Can you work these out from the model? Positions are in its coordinate system, mm. Face numbers are marked on the shaded views. A direction names the side the tool comes from. Give positions to 0.01 mm unless a question says otherwise; leave off trailing zeros. Order: outer loops, then holes, each group sorted by start corner. A loop starts at its lowest first (then second) coordinate and runs counter-clockwise, first axis right, second up. Notation, with made-up numbers: M 82,26.5 L 125,26.5 A22 cw 125,34.5 Z; hole C 24,-11.75 d2. An arc over 180 degrees is marked long. One line per question, with ' | ' between items. Start each with the question number.
1) If we section it at C-C, the plane y = 24: Please give me the cut outline in (x, z).
2) Please list where these lines run through material, in increasing order: line 1 along Z through (x, y) = (147, 0.75); line 2 along X through (y, z) = (1.15, -40.5); line 3 along Z through (x, y) = (34, 52). Write a range as [from, to].
3) If we section it at A-A, the plane z = -22: Please give me the cut outline in (x, y), plus the area to 3 significant figures.
4) I'm going to push flat-ended pins straight in: pin 1 Ø10 at (x, y) = (66.5, 10) entering from +Z; pin 2 Ø4 at (y, z) = (34.5, -45) entering from -X; pin 3 Ø3.5 at (x, z) = (107.5, -44.5) entering from -Y. Where does each tip first touch, or does it pass through?
5) Thinking about a two-plate mould opening in Z: for the marked faces 1, 2 and 3, which applies, +Z half, -Z half, draft (parallel to the pull), parting line (faces both ways), or undercut?
6) If we section it at D-D, the plane x = 107.5: Please give me the cut outline in (y, z), plus the area to 3 significant figures.
7) For the marked faces 4, 5 and 6, which set-ups out of +Z, -Z, +X, -X, +Y, -Y let a thin tool reach every point of the face, with its end or its side?
8) If we section it at B-B, the plane x = 87: Please give me the cut outline in (y, z).
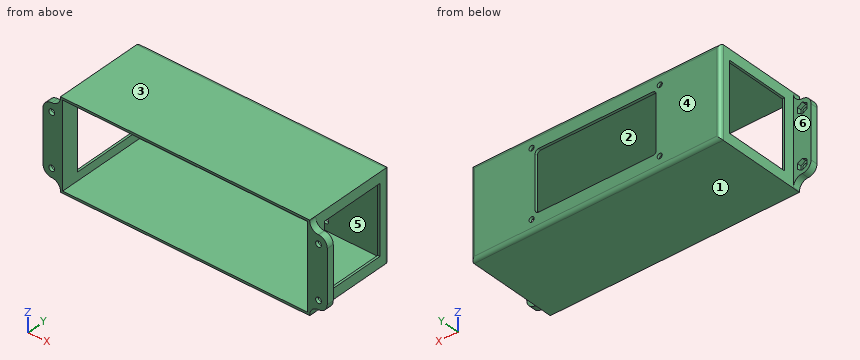
```python
from build123d import *

# Parameters (mm, degrees)
SKETCH1_W                 = 142
SKETCH1_H                 = 51
BOSS_EXTRUDE1_DEPTH       = 53
SHELL1_T                  = -1.25
SHELL1_THICKNESS_2_FACE_W = 48.5
SHELL1_THICKNESS_2_FACE_H = 139.5
SHELL1_THICKNESS_2_DEPTH  = 0.25
SKETCH2_W                 = 10
SKETCH2_H                 = 40
SKETCH2_R                 = 1.65
BOSS_EXTRUDE2_DEPTH       = 4
SKETCH3_W                 = 39
SKETCH3_H                 = 37
CUT_EXTRUDE1_DEPTH        = 169.860889492
CUT_EXTRUDE2_DEPTH        = 2.3
FILLET2_START             = -1
FILLET2_DEPTH             = 5
FILLET2_2_DEPTH           = 4
SKETCH5_R                 = 1.45
CUT_EXTRUDE3_DEPTH        = 169.860889492
SKETCH7_W                 = 69
SKETCH7_H                 = 34
CUT_EXTRUDE4_DEPTH        = 169.860889492
FILLET6_R                 = 2
FILLET7_R                 = 2


with BuildPart() as part:
    # Sketch1 → Boss-Extrude1 (new body)
    with BuildSketch(Plane(origin=(0, 0, 0), x_dir=(1, 0, 0), z_dir=(0, 1, 0))):
        with Locations((71, 25.5)):
            Rectangle(SKETCH1_W, SKETCH1_H)
    extrude(amount=BOSS_EXTRUDE1_DEPTH)

    # Shell1
    shell1_openings = [part.faces().sort_by_distance(p)[0] for p in [
        (71, 0, -25.5),
    ]]
    offset(amount=SHELL1_T, openings=shell1_openings, kind=Kind.INTERSECTION)

    # Shell1 thickness 2 face (on inner face of the shell) → Shell1 thickness 2 (add)
    with BuildSketch(Plane(origin=(71, 51.75, -25.5), x_dir=(0, 0, 1), z_dir=(0, 1, 0))):
        Rectangle(SHELL1_THICKNESS_2_FACE_W, SHELL1_THICKNESS_2_FACE_H)
    extrude(amount=-SHELL1_THICKNESS_2_DEPTH)

    # Sketch2 → Boss-Extrude2 (add)
    # profile 1 of 2: a face of its own
    with BuildSketch(Plane.XZ):
        with Locations((147, -25.5)):
            Rectangle(SKETCH2_W, SKETCH2_H)
        with Locations(Location((147, -40.5, 0), (0, 0, 270))):
            Circle(SKETCH2_R, mode=Mode.SUBTRACT)
        with Locations(Location((147, -10.5, 0), (0, 0, 270))):
            Circle(SKETCH2_R, mode=Mode.SUBTRACT)
    # profile 2 of 2: a face of its own
    with BuildSketch(Plane.XZ):
        with Locations((-5, -25.5)):
            Rectangle(SKETCH2_W, SKETCH2_H)
        with Locations(Location((-5, -40.5, 0), (0, 0, 270))):
            Circle(SKETCH2_R, mode=Mode.SUBTRACT)
        with Locations(Location((-5, -10.5, 0), (0, 0, 270))):
            Circle(SKETCH2_R, mode=Mode.SUBTRACT)
    extrude(amount=-BOSS_EXTRUDE2_DEPTH)

    # Sketch3 → Cut-Extrude1 (cut, through all)
    with BuildSketch(Plane(origin=(142, 0, 0), x_dir=(0, 0, -1), z_dir=(1, 0, 0))):
        with Locations((25.5, 28.5)):
            Rectangle(SKETCH3_W, SKETCH3_H)
    extrude(amount=-CUT_EXTRUDE1_DEPTH, mode=Mode.SUBTRACT)

    # Sketch4 → Cut-Extrude2 (cut)
    with BuildSketch(Plane(origin=(0, 4, 0), x_dir=(1, 0, 0), z_dir=(0, 1, 0))):
        Polygon((-5, 43.675426481), (-7.75, 42.08771324), (-7.75, 38.91228676), (-5, 37.324573519), (-2.25, 38.91228676), (-2.25, 42.08771324), align=None)
        Polygon((-5, 13.675426481), (-7.75, 12.08771324), (-7.75, 8.91228676), (-5, 7.324573519), (-2.25, 8.91228676), (-2.25, 12.08771324), align=None)
        Polygon((147, 43.675426481), (144.25, 42.08771324), (144.25, 38.91228676), (147, 37.324573519), (149.75, 38.91228676), (149.75, 42.08771324), align=None)
        Polygon((147, 13.675426481), (144.25, 12.08771324), (144.25, 8.91228676), (147, 7.324573519), (149.75, 8.91228676), (149.75, 12.08771324), align=None)
    extrude(amount=-CUT_EXTRUDE2_DEPTH, mode=Mode.SUBTRACT)

    # Fillet2: read off the stored shape, not the designer's step
    # Fillet2 outline → Fillet2 (cut)
    with BuildSketch(Plane(origin=(0, 0, 0), x_dir=(1, 0, 0), z_dir=(0, 1, 0)).offset(FILLET2_START)):
        with BuildLine():
            Line((-10, 5.5), (-5, 5.5))
            ThreePointArc((-5, 5.5), (-8.535533906, 6.964466094), (-10, 10.5))
            Line((-10, 10.5), (-10, 5.5))
        make_face()
        with BuildLine():
            Line((-10, 45.5), (-10, 40.5))
            ThreePointArc((-10, 40.5), (-8.535533906, 44.035533906), (-5, 45.5))
            Line((-5, 45.5), (-10, 45.5))
        make_face()
        with BuildLine():
            ThreePointArc((152, 10.5), (150.535533906, 6.964466094), (147, 5.5))
            Line((147, 5.5), (152, 5.5))
            Line((152, 5.5), (152, 10.5))
        make_face()
        with BuildLine():
            ThreePointArc((147, 45.5), (150.535533906, 44.035533906), (152, 40.5))
            Line((152, 40.5), (152, 45.5))
            Line((152, 45.5), (147, 45.5))
        make_face()
    extrude(amount=FILLET2_DEPTH, mode=Mode.SUBTRACT)

    # Fillet2 2 outline → Fillet2 2 (add)
    with BuildSketch(Plane(origin=(0, 0, 0), x_dir=(1, 0, 0), z_dir=(0, 1, 0))):
        with BuildLine():
            Line((0, 5.5), (-5, 5.5))
            ThreePointArc((-5, 5.5), (-1.464466094, 4.035533906), (0, 0.5))
            Line((0, 0.5), (0, 5.5))
        make_face()
        with BuildLine():
            Line((-5, 45.5), (0, 45.5))
            Line((0, 45.5), (0, 50.5))
            ThreePointArc((0, 50.5), (-1.464466094, 46.964466094), (-5, 45.5))
        make_face()
        with BuildLine():
            ThreePointArc((142, 0.5), (143.464466094, 4.035533906), (147, 5.5))
            Line((147, 5.5), (142, 5.5))
            Line((142, 5.5), (142, 0.5))
        make_face()
        with BuildLine():
            Line((142, 50.5), (142, 45.5))
            Line((142, 45.5), (147, 45.5))
            ThreePointArc((147, 45.5), (143.464466094, 46.964466094), (142, 50.5))
        make_face()
    extrude(amount=FILLET2_2_DEPTH)

    # Sketch5 → Cut-Extrude3 (cut, through all)
    with BuildSketch(Plane(origin=(0, 53, 0), x_dir=(1, 0, 0), z_dir=(0, 1, 0))):
        with Locations(Location((34.5, 44.5, 0), (0, 0, 270))):
            Circle(SKETCH5_R)
        with Locations(Location((34.5, 6.5, 0), (0, 0, 270))):
            Circle(SKETCH5_R)
        with Locations(Location((107.5, 6.5, 0), (0, 0, 270))):
            Circle(SKETCH5_R)
        with Locations(Location((107.5, 44.5, 0), (0, 0, 270))):
            Circle(SKETCH5_R)
    extrude(amount=-CUT_EXTRUDE3_DEPTH, mode=Mode.SUBTRACT)

    # Sketch7 → Cut-Extrude4 (cut, through all)
    with BuildSketch(Plane(origin=(0, 53, 0), x_dir=(1, 0, 0), z_dir=(0, 1, 0))):
        with Locations((71, 25.5)):
            Rectangle(SKETCH7_W, SKETCH7_H)
    extrude(amount=-CUT_EXTRUDE4_DEPTH, mode=Mode.SUBTRACT)

    # Fillet6
    fillet6_edges = [part.edges().sort_by_distance(p)[0] for p in [
        (36.5, 52.25, -8.5),
        (36.5, 52.25, -42.5),
        (105.5, 52.25, -42.5),
        (105.5, 52.25, -8.5),
    ]]
    fillet(fillet6_edges, radius=FILLET6_R)

    # Fillet7
    fillet7_edges = [part.edges().sort_by_distance(p)[0] for p in [
        (142, 53, -25.5),
        (71, 53, -51),
        (0, 53, -25.5),
        (71, 53, 0),
    ]]
    fillet(fillet7_edges, radius=FILLET7_R)


solid = part.part
```
Results found:
1) outline: M 0,-51 L 142,-51 L 142,-45 L 140.75,-45 L 140.75,-49.75 L 1.25,-49.75 L 1.25,-45 L 0,-45 Z; M 0,-6 L 1.25,-6 L 1.25,-1.25 L 140.75,-1.25 L 140.75,-6 L 142,-6 L 142,0 L 0,0 Z
2) line 1: z = [-45.5, -42.15], [-38.85, -12.15], [-8.85, -5.5] | line 2: x = [-10, -6.65], [-3.35, 1.25], [140.75, 145.35], [148.65, 152] | line 3: z = [-50.73, -45.86], [-43.14, -7.86], [-5.14, -0.27]
3) outline: M -10,0 L 1.25,0 L 1.25,10 L 0,10 L 0,4 L -10,4 Z; M 0,47 L 1.25,47 L 1.25,51.5 L 36.5,51.5 L 36.5,53 L 2,53 A2 ccw 0,51 Z; M 105.5,51.5 L 140.75,51.5 L 140.75,47 L 142,47 L 142,51 A2 ccw 140,53 L 105.5,53 Z; M 140.75,0 L 152,0 L 152,4 L 142,4 L 142,10 L 140.75,10 Z | area: 224 mm²
4) pin 1: stops at z = 0 | pin 2: stops at x = 0 | pin 3: stops at y = 51.5
5) face 1: -Z half | face 2: undercut | face 3: +Z half
6) outline: M 0,-51 L 51,-51 A2 ccw 53,-49 L 53,-45.95 L 51.5,-45.95 L 51.5,-49.75 L 0,-49.75 Z; M 0,-1.25 L 51.5,-1.25 L 51.5,-5.05 L 53,-5.05 L 53,-2 A2 ccw 51,0 L 0,0 Z; M 51.5,-43.05 L 53,-43.05 L 53,-7.95 L 51.5,-7.95 Z | area: 195 mm²
7) face 4: +Z, -Z, +X, -X, +Y | face 5: -Y | face 6: +Z, -Z, -X, +Y
8) outline: M 0,-51 L 51,-51 A2 ccw 53,-49 L 53,-42.5 L 51.5,-42.5 L 51.5,-49.75 L 0,-49.75 Z; M 0,-1.25 L 51.5,-1.25 L 51.5,-8.5 L 53,-8.5 L 53,-2 A2 ccw 51,0 L 0,0 Z
